Design review of the part built by this model. Coordinates are the model's own, in mm. Face numbers are marked on the shaded views. A direction names the side the tool comes from. Give positions to 0.01 mm unless a question says otherwise; leave off trailing zeros. Write each loop counter-clockwise with the first axis right and the second up, starting at its lowest first coordinate (ties: lowest second). Pieces come first, ordered by that corner, then holes. Notation, with made-up numbers: (50.25, -6.75) -> (95.25, -6.75) arc R20 cw to (95.25, -1.75) -> close; hole circle Ø11 at (-39.5, 80.5). An arc over 180 degrees is marked (long way). Answer as a JSON object with one key per item and string values.
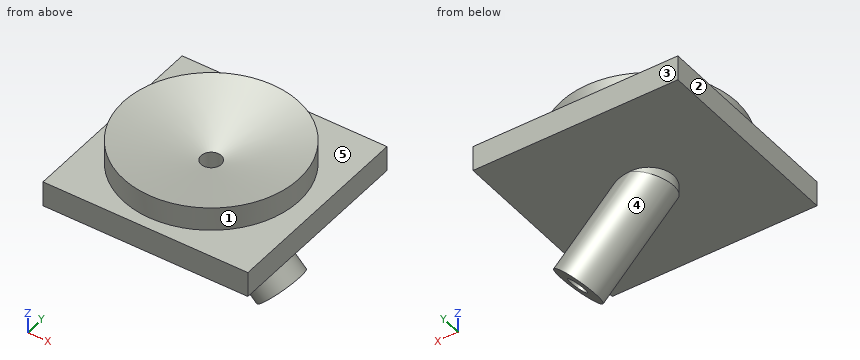
```python
from build123d import *

# Parameters (mm, degrees)
SKETCH7_R           = 1.475
SKETCH10_W          = 12.15
SKETCH10_H          = 11.8
BOSS_EXTRUDE1_DEPTH = 1.5
SKETCH5_R           = 0.6


with BuildPart() as part:
    # Sketch1 → Revolve1 (revolve)
    with BuildSketch(Plane(origin=(0, 0, 0), x_dir=(1, 0, 0), z_dir=(0, 1, 0))):
        Polygon((27.31279509, 4.648041847), (32.51279509, 4.648041847), (32.51279509, 1.748041847), (27.31279509, 3.148041847), align=None)
    revolve(axis=Axis((27.31279509, 0, -3.148041847), (0, 0, -1)))

    # Sweep2: sweep along a path in Sketch8
    with BuildLine(Plane(origin=(0, 0, 0), x_dir=(1, 0, 0), z_dir=(0, 1, 0))) as sweep2_path:
        Line((31.555435777, 8.890682534), (27.41279509, 4.648041847))
        Line((27.41279509, 4.648041847), (27.41279509, 3.648041847))
    # Sketch7 → Sweep2 (sweep)
    with BuildSketch(Plane(origin=(0, 0, -4.648041847), x_dir=(-1, 0, 0), z_dir=(0, 0, -1))):
        with Locations((-27.31279509, 0)):
            Circle(SKETCH7_R)
    sweep(path=sweep2_path.line, transition=Transition.RIGHT)

    # Sketch10 → Boss-Extrude1 (add)
    with BuildSketch(Plane(origin=(0, 0, -4.648041847), x_dir=(-1, 0, 0), z_dir=(0, 0, -1))):
        with Locations((-27.53779509, 0)):
            Rectangle(SKETCH10_W, SKETCH10_H)
    extrude(amount=-BOSS_EXTRUDE1_DEPTH)

    # Cut-Sweep2: sweep along a path in Sketch9
    with BuildLine(Plane(origin=(0, 0, 0), x_dir=(1, 0, 0), z_dir=(0, 1, 0))) as cut_sweep2_path:
        Line((27.41279509, 0), (27.41279509, 4.648041847))
        Line((27.41279509, 4.648041847), (31.655435777, 8.890682534))
    # Sketch5 → Cut-Sweep2 (sweep, cut)
    with BuildSketch(Plane.XY):
        with Locations((27.31279509, 0)):
            Circle(SKETCH5_R)
    sweep(path=cut_sweep2_path.line, transition=Transition.RIGHT, mode=Mode.SUBTRACT)


solid = part.part
```
(1) For the marked faces 1 and 2, list the 3-axis set-ups (+Z, -Z, +X, -X, +Y, -Y) from which the entire face can be reached by the end or side of a thin tool; tool diameter is ignored.
Here are the results:
{"face 1": "+Z", "face 2": "+Z, -Z, -X, +Y, -Y"}
(2) We need section A-A, the plane y = 0. State the section outline as (x, z) points, then the cut area to 3 significant figures.
Here are the results:
{"outline": "(21.46, -4.65) -> (25.84, -4.65) -> (25.84, -5.29) -> (30.43, -9.99) -> (31.11, -9.33) -> (26.71, -4.94) -> (26.71, -2.99) -> (22.11, -1.75) -> (22.11, -3.15) -> (21.46, -3.15) -> close; (27.91, -4.44) -> (31.96, -8.49) -> (32.54, -7.93) -> (29.33, -4.65) -> (33.61, -4.65) -> (33.61, -3.15) -> (32.51, -3.15) -> (32.51, -1.75) -> (27.91, -2.99) -> close", "area": "34.0 mm²"}
(3) For line 1 along Y through (x, z) = (28.5, -5.75); line 2 along Y through (x, z) = (30.75, -7.5); line 3 along X through (y, z) = (-0.25, -4), list the stretches that pass through material, from the lowest coordinate up.
Here are the results:
{"line 1": "y = -1.47 to -0.59, 0.59 to 1.47", "line 2": "y = -1.39 to -0.4, 0.4 to 1.39", "line 3": "x = 21.46 to 26.77, 27.86 to 33.61"}
(4) Clearance check with flat-ended pins moving along their axes: pin 1 (1 mm diameter, centred on x = 27.5, y = -3, fed in from +Z); pin 2 (1.4 mm diameter, centred on x = 27.31, y = 0, fed in from -Z); pin 3 (3.5 mm diameter, centred on x = 30.5, y = -2.5, fed in from -Z). State where each tip first meets the part, or that it passes through.
Here are the results:
{"pin 1": "stops at z = -2.2", "pin 2": "stops at z = -7.51", "pin 3": "stops at z = -9.85"}
(5) The part is to be moulded in two halves that separate along Z. For the marked faces 3, 4 and 5, say which applies: +Z half, -Z half, draft (parallel to the pull), parting line (faces both ways), or undercut.
Here are the results:
{"face 3": "draft", "face 4": "undercut", "face 5": "+Z half"}
(6) We need section B-B, the plane x = 30.75. Give the number of separate pieces and of enclosed holes in the cut face, then the cut area to 3 significant figures.
Here are the results:
{"separate pieces": "2", "enclosed holes": "1", "area": "33.5 mm²"}
